Verification items for the finished model (mm, model axes). A direction names the side the tool comes from. Give positions to 0.01 mm unless a question says otherwise; leave off trailing zeros. Answer in a Markdown table with one row per item.
```python
from build123d import *

# Parameters (mm, degrees)
F0_W          = 38.1
F0_H          = 38.1
F1_DEPTH      = 444.5
F5_DEPTH      = 19.0510001
F5_DEPTH_BACK = 19.0510001


with BuildPart() as f1:
    # F0 (on Top) → F1 (new body, symmetric)
    with BuildSketch(Plane.XY):
        Rectangle(F0_W, F0_H)
    extrude(amount=F1_DEPTH, both=True)

    # F2 (on Front) → F3 (revolve, cut)
    with BuildSketch(Plane.XZ):
        with BuildLine():
            add(Edge.make_bspline(
                [(11.5527668968, 0), (10.046800866, 28.4893312995), (9.1715674295, 80.9977363485), (5.0395663967, 129.2134805839), (12.9611159905, 184.4131507626), (-2.0989746226, 223.9534673168), (15.4149563286, 238.300591961), (19.05, 269.2452967167)],
                knots=[0, 0, 0, 0, 0.2471585757, 0.4397166911, 0.6422654444, 0.8019346241, 1, 1, 1, 1], degree=3))
            add(Edge.make_bspline(
                [(11.5527668968, 0), (10.046800866, -28.4893312995), (9.1715674295, -80.9977363485), (5.0395663967, -129.2134805839), (12.9611159905, -184.4131507626), (-2.0989746226, -223.9534673168), (15.4149563286, -238.300591961), (19.05, -269.2452967167)],
                knots=[0, 0, 0, 0, 0.2471585757, 0.4397166911, 0.6422654444, 0.8019346241, 1, 1, 1, 1], degree=3))
            Line((19.05, -269.2452967167), (67.6923958421, -269.2452967167))
            Line((67.6923958421, -269.2452967167), (67.6923958421, 269.2452967167))
            Line((67.6923958421, 269.2452967167), (19.05, 269.2452967167))
        make_face()
    revolve(axis=Axis((0, 0, 0), (0, 0, -1)), mode=Mode.SUBTRACT)

    # F4 (on Front) → F5 (cut, two sides)
    with BuildSketch(Plane.XZ) as f5_sk:
        Polygon((19.05, 444.5), (-19.05, 444.5), (19.05, 420.4699862058), align=None)
    extrude(amount=-F5_DEPTH, mode=Mode.SUBTRACT)
    extrude(f5_sk.sketch, amount=F5_DEPTH_BACK, mode=Mode.SUBTRACT)


solid = f1.part
```
Item 1: Release check for a two-part mould opening along Z. For faces 1 (the flat face through (-15, 15, -269.245)), 2 (the flat face through (0, 19.05, -356)), 3 (the flat face through (0, 0, -444.5)) record: released by +Z, released by -Z, zero draft, split by the parting line, or undercut.
Reported:
| item | result |
|---|---|
| face 1 | undercut |
| face 2 | zero draft |
| face 3 | released by -Z |
Item 2: Tool access check on faces 4 (the flat face through (15, 15, 269.245)), 5 (the flat face through (-14, -15, -269.245)), 6 (the flat face through (14, -15, 269.245)). Record the directions out of +Z, -Z, +X, -X, +Y, -Y that give a thin tool (end or side, any length) a straight path to the whole face; none if there is none.
Reported:
| item | result |
|---|---|
| face 4 | +X, +Y |
| face 5 | -X, -Y |
| face 6 | +X, -Y |
Item 3: Sectioned sample at A-A (y = 6.5). State how many separate pieces and enclosed holes the cut face has, and give its area (3 significant figures).
Reported:
| item | result |
|---|---|
| separate pieces | 3 |
| enclosed holes | 0 |
| area | 19,500 mm^2 |
Item 4: Go/stop test with flat-tipped pins: pin 1 (1.5 mm diameter, centred on x = 3.5, z = -49, fed in from +Y); pin 2 (8 mm diameter, centred on x = -12, y = -14.5, fed in from +Z); pin 3 (21 mm diameter, centred on x = 7, y = 8.5, fed in from +Z); pin 4 (21 mm diameter, centred on x = -11, y = 13, fed in from +Z). Record where each tip stops, or that it passes through.
Reported:
| item | result |
|---|---|
| pin 1 | stops at y = 9.25 |
| pin 2 | stops at z = 442.58 |
| pin 3 | stops at z = 434.69 |
| pin 4 | stops at z = 444.5 |
Item 5: Scan lines: L1, parallel to Z at x = -11.5, y = -1.5; L2, parallel to Z at x = 11.5, y = 10; L3, parallel to X at y = -0.5, z = -124. Record each from-to range of solid material in increasing order. Write a range as [from, to].
Reported:
| item | result |
|---|---|
| L1 | z = [-444.5, -238.61], [238.61, 439.74] |
| L2 | z = [-444.5, -249.32], [249.32, 425.23] |
| L3 | x = [-6.84, 6.84] |
